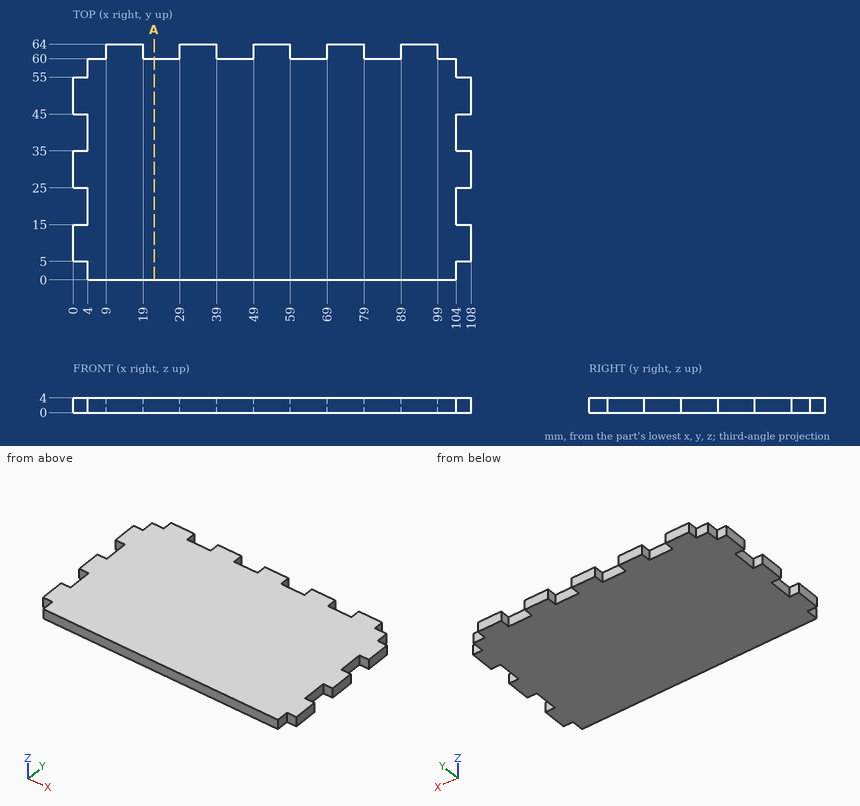
The figure shows three views and two pictorial views of one solid part (mm, origin at its lowest corner). Answer the questions. Round coordinates to 2 decimals unless told otherwise and drop trailing zeros. Order: outer loops, then holes, each group sorted by start corner. A loop starts at its lowest first (then second) coordinate and runs counter-clockwise, first axis right, second up. Notation, with made-up numbers: (60.5, 33.5) - (112.5, 33.5) arc R9 cw to (112.5, 37.5) - close; hole circle Ø6 at (-28.5, 15). An arc over 180 degrees is marked (long way). Write item = value, one per line. Start each with the question number.
1) Straight lines are drawn through the part: L1, parallel to X at y = 61.5, z = 2.85; L2, parallel to Y at x = 22.5, z = 1.9; L3, parallel to X at y = 22, z = 2.45. For each, find the intervals that lie inside material, in ascending order.
2) Section A-A, the plane x = 22 is taken. Write down the section's boundary in (y, z).
3) Given pin 1 (1.2 mm diameter, centred on x = 102.5, z = 1, fed in from +Y); pin 2 (1.2 mm diameter, centred on y = 61, z = 3, fed in from +X); pin 3 (1.2 mm diameter, centred on x = 105, z = 1.5, fed in from +Y), each flat-ended and moving along its own axis, determine where each tip first touches the part or whether it passes through.
Results list:
q1.L1 = 9 to 19, 29 to 39, 49 to 59, 69 to 79, 89 to 99
q1.L2 = 0 to 60
q1.L3 = 4 to 104
q2.outline = (0, 0) - (60, 0) - (60, 4) - (0, 4) - close
q3.pin_1 = 60
q3.pin_2 = 99
q3.pin_3 = 55
